```python
from build123d import *

# Parameters (mm, degrees)
DODANIE_WYCI_GNI_CIE1_DEPTH         = 45
DODANIE_WYCI_GNI_CIE1_DEPTH_BACK    = 45
SZKIC1_W                            = 45
SZKIC1_H                            = 45
WYTNIJ_WYCI_GNI_CIE1_DEPTH          = 96.45941546
WYTNIJ_WYCI_GNI_CIE1_DEPTH_BACK     = 96.45941546
SZKIC2_W                            = 42.5
SZKIC2_H                            = 40
DODANIE_WYCI_GNI_CIE2_DEPTH         = 70
DODANIE_WYCI_GNI_CIE2_DEPTH_BACK    = 2.5
SZKIC3_W                            = 45
SZKIC3_H                            = 100
SZKIC4_W                            = 40
SZKIC4_H                            = 70
WYTNIJ_WYCI_GNI_CIE2_DEPTH          = 144.461667354
SZKIC5_R                            = 8
WYTNIJ_WYCI_GNI_CIE4_DEPTH          = 90
ZAOKR_GLENIE2_R                     = 1
ZAOKR_GLENIE3_R                     = 1
SZKIC9_W                            = 4
SZKIC9_H                            = 45
OTWORY_USTALAJ_CE_8_0MM1_AT_2_COUNT = 2
OTWORY_USTALAJ_CE_8_0MM1_AT_2_PITCH = 22.5
OTWORY_USTALAJ_CE_8_0MM1_AT_3_COUNT = 2
OTWORY_USTALAJ_CE_8_0MM1_AT_3_PITCH = 45
SZKIC13_W                           = 4
SZKIC13_H                           = 145
OTWORY_USTALAJ_CE_8_0MM3_AT_2_COUNT = 2
OTWORY_USTALAJ_CE_8_0MM3_AT_2_PITCH = 45
DODANIE_WYCI_GNI_CIE3_DEPTH         = 1.5
DODANIE_WYCI_GNI_CIE3_DEPTH_BACK    = 1.5
ZAOKR_GLENIE4_R                     = 1.5


with BuildPart() as part:
    # Szkic1 → Dodanie-wyci_gni_cie1 (new, two sides: drawn at the far end of the back side and taken through both)
    with BuildSketch(Plane(origin=(0, 0, 0), x_dir=(0, 0, -1), z_dir=(1, 0, 0)).offset(-DODANIE_WYCI_GNI_CIE1_DEPTH_BACK)):
        Rectangle(SZKIC1_W, SZKIC1_H)
    extrude(amount=DODANIE_WYCI_GNI_CIE1_DEPTH + DODANIE_WYCI_GNI_CIE1_DEPTH_BACK)

    # Szkic2 → Wytnij-wyci_gni_cie1 (cut, two sides: drawn at the far end of the back side and taken through both)
    with BuildSketch(Plane.ZY.offset(45).offset(-WYTNIJ_WYCI_GNI_CIE1_DEPTH_BACK)):
        with Locations((-1.25, 0)):
            Rectangle(SZKIC2_W, SZKIC2_H)
    extrude(amount=WYTNIJ_WYCI_GNI_CIE1_DEPTH + WYTNIJ_WYCI_GNI_CIE1_DEPTH_BACK, mode=Mode.SUBTRACT)

    # Zaokr_glenie2
    zaokr_glenie2_edges = [part.edges().sort_by_distance(p)[0] for p in [
        (-45, 0, 22.5),
        (45, 22.5, 0),
        (45, 0, 22.5),
        (45, -22.5, 0),
        (-45, -22.5, 0),
        (0, 22.5, 22.5),
        (0, 22.5, -22.5),
        (-45, 22.5, 0),
    ]]
    fillet(zaokr_glenie2_edges, radius=ZAOKR_GLENIE2_R)

    # Szkic9 → Otwory ustalaj_ce _8.0mm1 (revolve, cut)
    with BuildSketch(Plane(origin=(-22.5, 0, 22.5), x_dir=(0, -1, 0), z_dir=(1, 0, 0))):
        with Locations((2, 22.5)):
            Rectangle(SZKIC9_W, SZKIC9_H)
    otwory_ustalaj_ce_8_0mm1 = revolve(axis=Axis((-22.5, 0, 28.85), (0, 0, -1)), mode=Mode.SUBTRACT)

    # Otwory ustalaj_ce _8.0mm1 at 2: Otwory ustalaj_ce _8.0mm1 ×2
    with Locations(*[(i * OTWORY_USTALAJ_CE_8_0MM1_AT_2_PITCH, 0, 0) for i in range(1, OTWORY_USTALAJ_CE_8_0MM1_AT_2_COUNT)]):
        add(otwory_ustalaj_ce_8_0mm1, mode=Mode.SUBTRACT)

    # Otwory ustalaj_ce _8.0mm1 at 3: Otwory ustalaj_ce _8.0mm1 ×2
    with Locations(*[(i * OTWORY_USTALAJ_CE_8_0MM1_AT_3_PITCH, 0, 0) for i in range(1, OTWORY_USTALAJ_CE_8_0MM1_AT_3_COUNT)]):
        add(otwory_ustalaj_ce_8_0mm1, mode=Mode.SUBTRACT)

    # Szkic13 → Otwory ustalaj_ce _8.0mm3 (revolve, cut)
    with BuildSketch(Plane(origin=(22.5, 22.5, 0), x_dir=(0, 0, 1), z_dir=(1, 0, 0))):
        with Locations((2, 72.5)):
            Rectangle(SZKIC13_W, SZKIC13_H)
    otwory_ustalaj_ce_8_0mm3 = revolve(axis=Axis((22.5, 28.85, 0), (0, -1, 0)), mode=Mode.SUBTRACT)

    # Otwory ustalaj_ce _8.0mm3 at 2: Otwory ustalaj_ce _8.0mm3 ×2
    with Locations(*[(-i * OTWORY_USTALAJ_CE_8_0MM3_AT_2_PITCH, 0, 0) for i in range(1, OTWORY_USTALAJ_CE_8_0MM3_AT_2_COUNT)]):
        add(otwory_ustalaj_ce_8_0mm3, mode=Mode.SUBTRACT)



with BuildPart() as body_2:
    # Szkic3 → Dodanie-wyci_gni_cie2 (new, two sides: drawn at the far end of the back side and taken through both)
    with BuildSketch(Plane.XY.offset(22.5).offset(-DODANIE_WYCI_GNI_CIE2_DEPTH_BACK)):
        with Locations((0, -72.5)):
            Rectangle(SZKIC3_W, SZKIC3_H)
    extrude(amount=DODANIE_WYCI_GNI_CIE2_DEPTH + DODANIE_WYCI_GNI_CIE2_DEPTH_BACK)

    # Szkic4 → Wytnij-wyci_gni_cie2 (cut, through all)
    with BuildSketch(Plane(origin=(0, -22.5, 0), x_dir=(1, 0, 0), z_dir=(0, 1, 0))):
        with Locations((0, -57.5)):
            Rectangle(SZKIC4_W, SZKIC4_H)
    extrude(amount=-WYTNIJ_WYCI_GNI_CIE2_DEPTH, mode=Mode.SUBTRACT)

    # Szkic5 → Wytnij-wyci_gni_cie4 (cut)
    with BuildSketch(Plane.ZY.offset(22.5)):
        Polygon((71.25, -89.5), (71.25, -122.5), (92.5, -122.5), (92.5, -22.5), (37.5, -22.5), align=None)
        with Locations(Location((56.25, -106, 0), (0, 0, 270))):
            Circle(SZKIC5_R)
    extrude(amount=-WYTNIJ_WYCI_GNI_CIE4_DEPTH, mode=Mode.SUBTRACT)

    # Zaokr_glenie3
    zaokr_glenie3_edges = [body_2.edges().sort_by_distance(p)[0] for p in [
        (22.5, -72.5, 20),
        (22.5, -98, 56.25),
        (-22.5, -98, 56.25),
        (-22.5, -72.5, 20),
        (-22.5, -56, 54.375),
        (22.5, -56, 54.375),
        (-22.5, -106, 71.25),
        (22.5, -106, 71.25),
        (-22.5, -22.5, 28.75),
        (22.5, -22.5, 28.75),
        (22.5, -122.5, 45.625),
        (-22.5, -122.5, 45.625),
        (0, -122.5, 20),
    ]]
    fillet(zaokr_glenie3_edges, radius=ZAOKR_GLENIE3_R)


with BuildPart() as part_1:
    add(part.part)

    add(body_2.part)  # Dodanie-wyci_gni_cie3 merges body 2
    # Szkic14 → Dodanie-wyci_gni_cie3 (add, two sides: drawn at the far end of the back side and taken through both)
    with BuildSketch(Plane.ZY.offset(-DODANIE_WYCI_GNI_CIE3_DEPTH_BACK)):
        Polygon((20, -121.5), (-22.5, -22.5), (20, -22.5), align=None)
    extrude(amount=DODANIE_WYCI_GNI_CIE3_DEPTH + DODANIE_WYCI_GNI_CIE3_DEPTH_BACK)

    # Zaokr_glenie4
    zaokr_glenie4_edges = [part_1.edges().sort_by_distance(p)[0] for p in [
        (1.5, -72, -1.25),
        (-1.5, -72, -1.25),
    ]]
    fillet(zaokr_glenie4_edges, radius=ZAOKR_GLENIE4_R - 0.0001)  # a hair under: the kernel refuses the full size


solid = part_1.part
```
Here's how the part is built. I have some questions about the finished solid (model axes, mm). A direction names the side the tool comes from. Round coordinates to 2 decimals unless told otherwise and drop trailing zeros. Write each loop counter-clockwise with the first axis right and the second up, starting at its lowest first coordinate (ties: lowest second). Pieces come first, ordered by that corner, then holes.
Q1. If we section it at C-C on x = 7: Write out the boundary of the cut face in (y, z).
Q2. If we section it at D-D on x = -24.5: Write out the boundary of the cut face in (y, z), plus the area to 3 significant figures.
Q3. If we section it at B-B on y = 0: Write out the boundary of the cut face in (x, z).
Q4. If we section it at A-A on z = 27: Write out the boundary of the cut face in (x, y).
Q5. Will these pins go through, and if not, where does the flat tip stop? P1, Ø4, axis at x = -29, y = -14.5, coming from the -Z side; P2, Ø24.5, axis at y = -48, z = 36, coming from the -X side; P3, Ø13, axis at x = 22.5, z = 0, coming from the +Y side; P4, Ø17, axis at x = 7, y = -71, coming from the -Z side.
Q6. Which directions (+Z, -Z, +X, -X, +Y, -Y) give clear straight access to the entire face, cutting with the end or side of a thin tool? Please do faces 1 (the flat face through (1, -20, -2)), 2 (the cylindrical face through (-26.466, 0.521, 21.232)), 3 (the flat face through (-20, -83, 42)).
Q7. Please list where these lines run through material, in increasing order: probe 1 along X at (y, z) = (21.05, 0); probe 2 along Y at (x, z) = (-5, 3.5).
Q8. If we mould it in two halves opening along Z, with no side actions, what happens to faces 4 (the flat face through (-1.5, -59, 4)), 5 (the cylindrical face through (20.74, -110.301, 62.996)), 6 (the cylindrical face through (1.05, -71.14, -1.15))? For each: +Z half, -Z half, draft (parallel to the pull), parting line (faces both ways), or undercut.
Answer below:
1. outline: (-122.5, 21) arc R1 ccw to (-121.5, 20) - (-22.5, 20) - (-22.5, -22.5) - (-20, -22.5) - (-20, 20) - (20, 20) - (20, -22.5) - (21.5, -22.5) arc R1 ccw to (22.5, -21.5) - (22.5, 21.5) arc R1 ccw to (21.5, 22.5) - (-122.5, 22.5) - close
2. outline: (-22.5, -22.5) - (-20, -22.5) - (-20, -3.46) - (-22.5, -3.46) - close; (-22.5, 3.46) - (-20, 3.46) - (-20, 20) - (-3.46, 20) - (-3.46, 22.5) - (-22.5, 22.5) - close; (3.46, 20) - (20, 20) - (20, 3.46) - (22.5, 3.46) - (22.5, 21.5) arc R1 ccw to (21.5, 22.5) - (3.46, 22.5) - close; (20, -22.5) - (21.5, -22.5) arc R1 ccw to (22.5, -21.5) - (22.5, -3.46) - (20, -3.46) - close
2. area: 273 mm2
3. outline: (-45, 20) - (-26.5, 20) - (-26.5, 22.5) - (-44, 22.5) arc R1 ccw to (-45, 21.5) - close; (-18.5, 20) - (-4, 20) - (-4, 22.5) - (-18.5, 22.5) - close; (4, 20) - (18.5, 20) - (18.5, 22.5) - (4, 22.5) - close; (26.5, 20) - (45, 20) - (45, 21.5) arc R1 ccw to (44, 22.5) - (26.5, 22.5) - close
4. outline: (-22.5, -121.5) arc R1 ccw to (-21.5, -122.5) - (-20, -122.5) - (-20, -22.5) - (-21.5, -22.5) arc R1 ccw to (-22.5, -23.5) - close; (20, -122.5) - (21.5, -122.5) arc R1 ccw to (22.5, -121.5) - (22.5, -23.5) arc R1 ccw to (21.5, -22.5) - (20, -22.5) - close
5. P1: stops at z = 20
5. P2: stops at x = -22.5
5. P3: stops at y = 22.5
5. P4: stops at z = -3.94
6. face 1: -Z, +X, -X
6. face 2: +Z, -Z
6. face 3: +Z, +Y, -Y
7. probe 1: x = -45 to -26.5, -18.5 to 18.5, 26.5 to 45
7. probe 2: y = -22.5 to -20, 20 to 22.5
8. face 4: draft
8. face 5: undercut
8. face 6: -Z half
